Source: CAD feature listing. Evaluate the final solid. Frame: model axes, mm. Round coordinates to 2 decimals unless told otherwise and drop trailing zeros. Write each loop counter-clockwise with the first axis right and the second up, starting at its lowest first coordinate (ties: lowest second). Pieces come first, ordered by that corner, then holes. Notation, with made-up numbers: M 10,64.5 L 47,64.5 A33 cw 47,95.5 Z; hole C -35,39.5 d5. An arc over 180 degrees is marked long. Put each result on its own line as item: value. Start each with the question number.
```python
from build123d import *

# Parameters (mm, degrees)
SKETCH065_W     = 40
SKETCH065_H     = 40
PAD035_DEPTH    = 1220
SKETCH066_W     = 40
SKETCH066_H     = 40
POCKET020_DEPTH = 20
SKETCH067_R     = 5
POCKET021_DEPTH = 40.001


with BuildPart() as part:
    # Sketch065 → Pad035 (new body)
    with BuildSketch(Plane.XZ.offset(280)):
        with Locations((1200, 280)):
            Rectangle(SKETCH065_W, SKETCH065_H)
    extrude(amount=PAD035_DEPTH)

    # Sketch066 (on Face3 of Pad035) → Pocket020 (cut)
    with BuildSketch(Plane(origin=(0, 0, 260), x_dir=(1, 0, 0), z_dir=(0, 0, -1))):
        with Locations((1200, 1480)):
            Rectangle(SKETCH066_W, SKETCH066_H)
        with Locations((1200, 300)):
            Rectangle(SKETCH066_W, SKETCH066_H)
    extrude(amount=-POCKET020_DEPTH, mode=Mode.SUBTRACT)

    # Sketch067 (on Face1 of Pocket020) → Pocket021 (cut, through all)
    with BuildSketch(Plane(origin=(0, 0, 300), x_dir=(-1, 0, 0), z_dir=(0, 0, 1))):
        with Locations((-1200, 1480)):
            Circle(SKETCH067_R)
        with Locations((-1200, 300)):
            Circle(SKETCH067_R)
    extrude(amount=-POCKET021_DEPTH, mode=Mode.SUBTRACT)


with BuildPart() as part_1:
    # Clone015 placement: moved
    add(part.part.moved(Location((0, 0, 450))))


solid = part_1.part
```
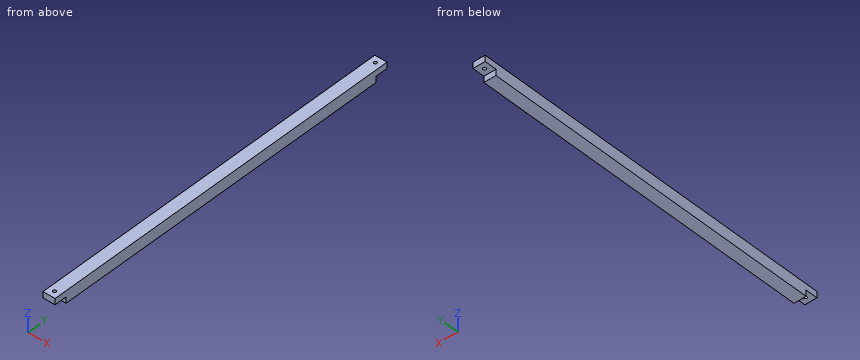
(1) Section query A-A (x = 1187.5). Return loops of the section in (y, z), and give its area (3 significant figures).
(2) Contact query for flat-ended pins moving along their axis: P1, Ø8, axis at x = 1200, y = -300, coming from the -Z side; P2, Ø20, axis at x = 1195, y = -1475.5, coming from the -Z side; P3, Ø6, axis at x = 1194, z = 724.5, coming from the +Y side; P4, Ø6, axis at x = 1192, z = 722, coming from the -Y side. Output: stop coordinate, or through.
(3) Section query B-B (z = 718). Return loops of the section in (x, y).
(4) Ray query, line 1 along Y through (x, z) = (1200, 736); line 2 along Y through (x, z) = (1201, 741.5); line 3 along X through (y, z) = (-300, 743.5). Return the intervals inside material, ascending.
Entries:
1. outline: M -1500,730 L -1460,730 L -1460,710 L -320,710 L -320,730 L -280,730 L -280,750 L -1500,750 Z
1. area: 47,200 mm2
2. P1: through
2. P2: z = 730
2. P3: y = -320
2. P4: y = -1460
3. outline: M 1180,-1460 L 1220,-1460 L 1220,-320 L 1180,-320 Z
4. line 1: -1500 to -1485, -1475 to -305, -295 to -280
4. line 2: -1500 to -1484.9, -1475.1 to -304.9, -295.1 to -280
4. line 3: 1180 to 1195, 1205 to 1220
